```python
from build123d import *

# Parameters (mm, degrees)
SKETCH1_W                      = 150
SKETCH1_H                      = 100
BASE_FLANGE1_DEPTH             = 1
EDGE_FLANGE1_STRIP_W           = 8
EDGE_FLANGE1_STRIP_H           = 1
EDGE_FLANGE1_STRIP_CUT_DEPTH   = 150
EDGE_FLANGE1_STRIP_2_W         = 8
EDGE_FLANGE1_STRIP_2_H         = 1
EDGE_FLANGE1_STRIP_CUT_2_DEPTH = 150
EDGE_FLANGE1_DEPTH             = 150
EDGE_FLANGE1_BEND_DEPTH        = 150
BREAK_CORNER1_START            = -51
BREAK_CORNER1_DEPTH            = 102
M4_CLEARANCE_HOLE1_D           = 4.8
M4_CLEARANCE_HOLE2_D           = 4.8


# Read off the part's stored shape, not the designer's step: Break-Corner1
# Sheet-metal steps are written as plain solids
with BuildPart() as part:
    # Sketch1 → Base-Flange1 (new body)
    with BuildSketch(Plane(origin=(0, 0, 0), x_dir=(1, 0, 0), z_dir=(0, 1, 0))):
        Rectangle(SKETCH1_W, SKETCH1_H)
    extrude(amount=-BASE_FLANGE1_DEPTH)

    # Edge-Flange1 strip (across the edge) → Edge-Flange1 strip cut (cut)
    with BuildSketch(Plane(origin=(-75, -1, -50), x_dir=(0, 0, 1), z_dir=(1, 0, 0))):
        with Locations((-2, -0.5)):
            Rectangle(EDGE_FLANGE1_STRIP_W, EDGE_FLANGE1_STRIP_H)
    extrude(amount=EDGE_FLANGE1_STRIP_CUT_DEPTH, mode=Mode.SUBTRACT)

    # Edge-Flange1 strip 2 (across the edge) → Edge-Flange1 strip cut 2 (cut)
    with BuildSketch(Plane(origin=(75, -1, 50), x_dir=(0, 0, -1), z_dir=(-1, 0, 0))):
        with Locations((-2, -0.5)):
            Rectangle(EDGE_FLANGE1_STRIP_2_W, EDGE_FLANGE1_STRIP_2_H)
    extrude(amount=EDGE_FLANGE1_STRIP_CUT_2_DEPTH, mode=Mode.SUBTRACT)

    # Edge-Flange1 section (across the edge) → Edge-Flange1 (add)
    with BuildSketch(Plane(origin=(-75, -1, -50), x_dir=(0, 0, 1), z_dir=(1, 0, 0))):
        with BuildLine():
            Line((-1, 2), (-1, 63))
            Line((-1, 63), (0, 63))
            Line((0, 63), (0, 2))
            ThreePointArc((0, 2), (0.585786438, 0.585786438), (2, 0))
            Line((2, 0), (2, -1))
            ThreePointArc((2, -1), (-0.121320344, -0.121320344), (-1, 2))
        make_face()
    extrude(amount=EDGE_FLANGE1_DEPTH)

    # Edge-Flange1 section 2 (across the edge) → Edge-Flange1 bend (add)
    with BuildSketch(Plane(origin=(75, -1, 50), x_dir=(0, 0, -1), z_dir=(-1, 0, 0))):
        with BuildLine():
            Line((-1, 2), (-1, 63))
            Line((-1, 63), (0, 63))
            Line((0, 63), (0, 2))
            ThreePointArc((0, 2), (0.585786438, 0.585786438), (2, 0))
            Line((2, 0), (2, -1))
            ThreePointArc((2, -1), (-0.121320344, -0.121320344), (-1, 2))
        make_face()
    extrude(amount=EDGE_FLANGE1_BEND_DEPTH)

    # Break-Corner1 outline → Break-Corner1 (cut)
    with BuildSketch(Plane.XY.offset(BREAK_CORNER1_START)):
        with BuildLine():
            Line((-75, -64), (-72, -64))
            ThreePointArc((-72, -64), (-74.121320344, -63.121320344), (-75, -61))
            Line((-75, -61), (-75, -64))
        make_face()
        with BuildLine():
            ThreePointArc((75, -61), (74.121320344, -63.121320344), (72, -64))
            Line((72, -64), (75, -64))
            Line((75, -64), (75, -61))
        make_face()
    extrude(amount=BREAK_CORNER1_DEPTH, mode=Mode.SUBTRACT)

    # M4 Clearance Hole1 (through all)
    with Locations(Plane(origin=(0, 0, -51), x_dir=(-1, 0, 0), z_dir=(0, 0, -1))):
        with Locations((-28, -54), (28, -54)):
            Hole(M4_CLEARANCE_HOLE1_D / 2)

    # M4 Clearance Hole2 (through all)
    with Locations(Plane(origin=(0, 0, 0), x_dir=(1, 0, 0), z_dir=(0, 1, 0))):
        with Locations((-65, 38), (-65, -38), (65, -38), (65, 38)):
            Hole(M4_CLEARANCE_HOLE2_D / 2)


solid = part.part
```
The model under review builds one solid part; all positions refer to its coordinate system, in mm. A direction names the side the tool comes from. Round coordinates to 2 decimals unless told otherwise and drop trailing zeros. Loops run counter-clockwise (first coordinate to the right, second up) from the corner with the lowest first, then second, coordinate; pieces in that order, holes last. Notation, with made-up numbers: (-1.5, -18.75) - (46.5, -18.75) arc R33 cw to (46.5, 11.25) - close; hole circle Ø9 at (51.25, 49.25). An arc over 180 degrees is marked (long way). Use a Markdown table: item, result. Add a question column.
Q1. Insertion check: pin 1 Ø7.5 at (x, z) = (-65, 38) entering from -Y. The pin has a flat end and moves straight along its axis. Give the tip position at first contact, or say it passes through.
Q2. Machinability: for faces 4 (the face through (-1, -34, -50)), 5 (the face through (1, -33, 51)), which of the approach directions +Z, -Z, +X, -X, +Y, -Y give a long, thin tool a straight path to every point of the face, cutting with its end or side? Answer none if there is none.
Q3. The part is to be moulded in two halves that separate along Y. For faces 1 (the face through (74.14, -63.1, -50.51)), 2 (the face through (63.89, -0.51, 40.13)), 3 (the face through (-26.89, -56.13, -50.49)), say which applies: pulls with the +Y half, pulls with the -Y half, needs draft (parallel to the pull), parting line crosses it, or undercut.
Q4. For probe 1 along X at (y, z) = (-0.6, 38); probe 2 along Z at (x, y) = (11, -51); probe 3 along Z at (x, y) = (-65, -0.35), list the stretches that pass through material, from the lowest coordinate up.
Q5. Add section C-C (x = 28). State the section outline as (y, z) points.
Q6. Add section A-A (y = -59). State the section outline as (x, z) points.
Q7. Add section D-D (x = 5.5). State the section outline as (y, z) points.
Q8. Add section B-B (z = -38). State the section outline as (x, y) points, plus the area to 3 significant figures.
Worked answers:
| question | item | result |
|---|---|---|
| 1 | pin 1 | y = -1 |
| 2 | face 4 | +X, -X, -Y |
| 2 | face 5 | +Z, +X, -X, +Y, -Y |
| 3 | face 1 | pulls with the -Y half |
| 3 | face 2 | needs draft |
| 3 | face 3 | undercut |
| 4 | probe 1 | -75 to -67.4, -62.6 to 62.6, 67.4 to 75 |
| 4 | probe 2 | -51 to -50, 50 to 51 |
| 4 | probe 3 | -49.41 to -40.4, -35.6 to 35.6, 40.4 to 49.41 |
| 5 | outline | (-64, -51) - (-56.4, -51) - (-56.4, -50) - (-64, -50) - close; (-64, 50) - (-56.4, 50) - (-56.4, 51) - (-64, 51) - close; (-51.6, -51) - (-3, -51) arc R3 ccw to (0, -48) - (0, 48) arc R3 ccw to (-3, 51) - (-51.6, 51) - (-51.6, 50) - (-3, 50) arc R2 cw to (-1, 48) - (-1, -48) arc R2 cw to (-3, -50) - (-51.6, -50) - close |
| 6 | outline | (-75, -51) - (75, -51) - (75, -50) - (-75, -50) - close; (-75, 50) - (75, 50) - (75, 51) - (-75, 51) - close |
| 7 | outline | (-64, -51) - (-3, -51) arc R3 ccw to (0, -48) - (0, 48) arc R3 ccw to (-3, 51) - (-64, 51) - (-64, 50) - (-3, 50) arc R2 cw to (-1, 48) - (-1, -48) arc R2 cw to (-3, -50) - (-64, -50) - close |
| 8 | outline | (-75, -1) - (-67.4, -1) - (-67.4, 0) - (-75, 0) - close; (-62.6, -1) - (62.6, -1) - (62.6, 0) - (-62.6, 0) - close; (67.4, -1) - (75, -1) - (75, 0) - (67.4, 0) - close |
| 8 | area | 140 mm² |
